from build123d import *

# Parameters (mm, degrees)
EXTRUDE_1_DEPTH          = 49
SKETCH_2_W               = 70
SKETCH_2_H               = 45
CUT_EXTRUDE_1_DEPTH      = 55.224494
CUT_EXTRUDE_1_TAPER      = 3
SKETCH_3_W               = 72
SKETCH_3_H               = 47
CUT_EXTRUDE_2_DEPTH      = 1
SKETCH_5_W               = 3
SKETCH_5_H               = 3
CUT_EXTRUDE_3_DEPTH      = 2
EXTRUDE_2_DEPTH          = 3
EXTRUDE_3_DEPTH          = 3
SKETCH_9_W               = 92.207980396
SKETCH_9_H               = 62.219536403
CUT_EXTRUDE_4_DEPTH      = 20
CUT_EXTRUDE_4_DEPTH_BACK = 32.556614873


with BuildPart() as part:
    # Sketch 1 → Extrude 1 (new body)
    with BuildSketch(Plane.XY):
        Polygon((16.715993843, 25.667879294), (20.215993843, -31.556614873), (87.215993843, -31.556614873), (90.715993843, 25.667879294), align=None)
    extrude(amount=EXTRUDE_1_DEPTH)

    # Sketch 2 → Cut-Extrude 1 (cut)
    with BuildSketch(Plane(origin=(0, 25.667879294, 0), x_dir=(1, 0, 0), z_dir=(0, 1, 0))):
        with Locations((53.715993843, -24.5)):
            Rectangle(SKETCH_2_W, SKETCH_2_H)
    extrude(amount=-CUT_EXTRUDE_1_DEPTH, taper=CUT_EXTRUDE_1_TAPER, mode=Mode.SUBTRACT)

    # Sketch 3 → Cut-Extrude 2 (cut)
    with BuildSketch(Plane(origin=(0, 25.667879294, 0), x_dir=(1, 0, 0), z_dir=(0, 1, 0))):
        with Locations((53.715993843, -24.5)):
            Rectangle(SKETCH_3_W, SKETCH_3_H)
    extrude(amount=-CUT_EXTRUDE_2_DEPTH, mode=Mode.SUBTRACT)

    # Sketch 5 → Cut-Extrude 3 (cut)
    with BuildSketch(Plane(origin=(20.006241746, 1.048482702, 0), x_dir=(0, 0, -1), z_dir=(0.998629535, 0.052335956, 0))):
        with Locations((-37.25, 21.151810576)):
            Rectangle(SKETCH_5_W, SKETCH_5_H)
        with Locations((-11.75, 21.206889344)):
            Rectangle(SKETCH_5_W, SKETCH_5_H)
    cut_extrude_3 = extrude(amount=-CUT_EXTRUDE_3_DEPTH, mode=Mode.SUBTRACT)

    # Sketch 6 → Extrude 2 (add)
    with BuildSketch(Plane.XY.offset(35.75)):
        Polygon((18.977745448, 20.673361155), (16.95854549, 21.70219492), (17.027722258, 20.57116477), align=None)
    extrude_2 = extrude(amount=EXTRUDE_2_DEPTH)

    # Sketch 7 → Extrude 3 (add)
    with BuildSketch(Plane(origin=(0, 0, 13.25), x_dir=(-1, 0, 0), z_dir=(0, 0, -1))):
        Polygon((-18.974862848, 20.728364439), (-17.024359652, 20.626142898), (-16.955165856, 21.757451456), align=None)
    extrude_3 = extrude(amount=EXTRUDE_3_DEPTH)

    # Mirror 2: Cut-Extrude 3, Extrude 2, Extrude 3 across plane
    add(cut_extrude_3.mirror(Plane(origin=(53.715993843, 0, 0), x_dir=(0, 0, 1), z_dir=(1, 0, 0))), mode=Mode.SUBTRACT)
    add(extrude_2.mirror(Plane(origin=(53.715993843, 0, 0), x_dir=(0, 0, 1), z_dir=(1, 0, 0))))
    add(extrude_3.mirror(Plane(origin=(53.715993843, 0, 0), x_dir=(0, 0, 1), z_dir=(1, 0, 0))))

    # Sketch 9 → Cut-Extrude 4 (cut, two sides)
    with BuildSketch(Plane(origin=(0, 0, 0), x_dir=(1, 0, 0), z_dir=(0, 1, 0))) as cut_extrude_4_sk:
        with Locations((56.409215525, -25.014933301)):
            Rectangle(SKETCH_9_W, SKETCH_9_H)
    extrude(amount=CUT_EXTRUDE_4_DEPTH, mode=Mode.SUBTRACT)
    extrude(cut_extrude_4_sk.sketch, amount=-CUT_EXTRUDE_4_DEPTH_BACK, mode=Mode.SUBTRACT)


solid = part.part
Model file for the job. Use its own axes, mm. A direction names the side the tool comes from. Give positions to 0.01 mm unless a question says otherwise; leave off trailing zeros. Use a Markdown table: item, result. Add a question column.
(1) Drop flat-ended pins along their axis: pin 1 Ø12 at (x, z) = (56, 35) entering from +Y; pin 2 Ø23.5 at (x, z) = (64.5, 35.5) entering from +Y; pin 3 Ø1.1 at (y, z) = (25, 28) entering from +X. Give the stop position or say it passes through.
(2) Mould opens along Y. For faces 4 (the flat face through (17.843, 23.673, 11.771)), 5 (the flat face through (51, 20, 48)), 6 (the flat face through (53, 23, 0)) say: +Y half, -Y half, draft (parallel to the pull), parting line (faces both ways), or undercut.
(3) Wall check: line 1 along Z through (x, y) = (39, 24.7); line 2 along X through (y, z) = (20.3, 33.5); line 3 along X through (y, z) = (23.65, 26.5). Give the ranges that are in metal, low to high.
(4) Tool access for faces 1 (the flat face through (89.586, 23.618, 37.271)), 2 (the flat face through (53.9, 25.668, 0.8)), 3 (the flat face through (53.5, 24.668, 1.8)): list every direction of +Z, -Z, +X, -X, +Y, -Y with a clear straight run to the whole face (end or side of a thin tool).
Filled sheet:
| question | item | result |
|---|---|---|
| 1 | pin 1 | through |
| 1 | pin 2 | y = 24.67 |
| 1 | pin 3 | x = 90.71 |
| 2 | face 4 | undercut |
| 2 | face 5 | -Y half |
| 2 | face 6 | draft |
| 3 | line 1 | 0 to 1, 48 to 49 |
| 3 | line 2 | 17.04 to 19, 88.43 to 90.39 |
| 3 | line 3 | 16.84 to 18.82, 88.61 to 90.59 |
| 4 | face 1 | none |
| 4 | face 2 | +Z, -Z, +X, -X, +Y |
| 4 | face 3 | +Y |
